```python
from build123d import *

# Parameters (mm, degrees)
PAD013_DEPTH    = 10
SKETCH065_W     = 4.5
SKETCH065_H     = 5.5
SKETCH065_W_2   = 3.4
SKETCH065_H_2   = 9
POCKET012_DEPTH = 7.2375310186


with BuildPart() as part:
    # Sketch064 → Pad013 (new body, symmetric)
    with BuildSketch(Plane.YZ):
        with BuildLine():
            ThreePointArc((-25.8475912574, 5.4708262373), (-29.159051684, -0.0593501339), (-30.5394960729, -6.355618405))
            ThreePointArc((-30.5394960729, -6.355618405), (-30.457390957, -6.658226438), (-30.2112344729, -6.8524424441))
            Line((-30.2112344729, -6.8524424441), (-29.3637121644, -7.1609153372))
            ThreePointArc((-29.3637121644, -7.1609153372), (-28.0255949556, -7.1024918781), (-27.1207148272, -6.1149885016))
            Line((-27.1207148272, -6.1149885016), (-23.4782003008, 3.8927379097))
            ThreePointArc((-23.4782003008, 3.8927379097), (-23.5115851346, 4.6573763148), (-24.0758727783, 5.1744506738))
            Line((-25.2946071344, 5.618033703), (-24.0758727783, 5.1744506738))
            ThreePointArc((-25.2946071344, 5.618033703), (-25.5942405308, 5.6313602812), (-25.8475912574, 5.4708262373))
        make_face()
    extrude(amount=PAD013_DEPTH, both=True)

    # Sketch065 (on Face6 of Pad013) → Pocket012 (cut, through all)
    with BuildSketch(Plane(origin=(0, -21.9828744359, 8.0011119583), x_dir=(0, 0.3420201433, 0.9396926208), z_dir=(0, 0.9396926208, -0.3420201433))):
        with Locations((-14.5220403435, 7.25)):
            Rectangle(SKETCH065_W, SKETCH065_H)
        with Locations((-14.5220403435, -7.25)):
            Rectangle(SKETCH065_W, SKETCH065_H)
        with Locations((-5.0720403435, 0)):
            Rectangle(SKETCH065_W_2, SKETCH065_H_2)
    extrude(amount=-POCKET012_DEPTH, mode=Mode.SUBTRACT)

    # SubtractivePipe003: sweep along a path in Sketch067
    with BuildLine(Plane.YZ.offset(4.5)) as subtractivepipe003_path:
        ThreePointArc((-25.6193920552, 5.7362457467), (-29.1630396012, -0.0694100418), (-30.5561005443, -6.7269214592))
    # Sketch066 (on DatumPlane) → SubtractivePipe003 (sweep, cut)
    with BuildSketch(Plane(origin=(4.5, -30.5394960729, -6.355618405), x_dir=(0, -0.9985433434, 0.0539554573), z_dir=(0, -0.0539554573, -0.9985433434))):
        Polygon((0, -0.025), (0, 0.025), (-0.0433012702, 0), align=None)
    subtractivepipe003 = sweep(path=subtractivepipe003_path.line, mode=Mode.SUBTRACT)

    # Mirrored003: SubtractivePipe003 across YZ
    add(subtractivepipe003.mirror(Plane.YZ), mode=Mode.SUBTRACT)


solid = part.part
```
Check sheet for the modelled part. Datum: model origin and axes. Units: mm. A direction names the side the tool comes from. Round coordinates to 2 decimals unless told otherwise and drop trailing zeros. Order: outer loops, then holes, each group sorted by start corner. A loop starts at its lowest first (then second) coordinate and runs counter-clockwise, first axis right, second up. Notation, with made-up numbers: (62.25, 44.5) - (117.25, 44.5) arc R9 ccw to (117.25, 60.5) - close; hole circle Ø6 at (-35, -22.5). An arc over 180 degrees is marked (long way). Answer as CSV lines item,"result". Start each with the question number.
1) Section check C-C (x = 4). Record the cut outline in (y, z), then the cut area to 3 significant figures.
2) Scan lines: probe 1 along X at (y, z) = (-25.5, 2.75); probe 2 along X at (y, z) = (-28.25, -3); probe 3 along Y at (x, z) = (-6.5, 3). Record each from-to range of solid material in increasing order.
3) Section check B-B (y = -24.75). Record the cut outline in (x, z).
4) Tool access check on faces 4 (the face through (4.5, -29, -5)), 5 (the face through (-4.5, -29, -5)), 6 (the face through (4.5, -25, 4)), 7 (the face through (-7.224, -28.249, 1.915)). Record the directions out of +Z, -Z, +X, -X, +Y, -Y that give a thin tool (end or side, any length) a straight path to the whole face; none if there is none.
5) Draft check along X on faces 1 (the face through (-0.06, -25.98, 2.25)), 2 (the face through (0.06, -28.04, -7.11)), 3 (the face through (-10, -27, 1)). Enter one of: +X half, -X half, draft (parallel to the pull), parting line (faces both ways), or undercut.
6) Section check A-A (x = 6.5). Record the cut outline in (y, z).
7) Depth check by flat-ended pin: pin 1 (4 mm diameter, centred on y = -28.5, z = -5.5, fed in from +X); pin 2 (2 mm diameter, centred on x = 2.5, y = -26.5, fed in from -Z); pin 3 (5 mm diameter, centred on x = -4.5, z = 1, fed in from +Y). Enter the tip coordinate at first touch or a pass-through.
Determined:
1,outline,"(-30.54, -6.36) arc R0.5 ccw to (-30.21, -6.85) - (-29.36, -7.16) arc R1.75 ccw to (-27.12, -6.11) - (-24.3, 1.64) - (-27.71, 2.88) arc R20 ccw to start"
1,area,"36.8 mm^2"
2,probe 1,"-10 to -4.5, 4.5 to 10"
2,probe 2,"-4.5 to 4.5"
2,probe 3,"-27.63 to -23.8"
3,outline,"(-10, 0.4) - (10, 0.4) - (10, 5.42) - (4.5, 5.42) - (4.5, 1.8) - (-4.5, 1.8) - (-4.5, 5.42) - (-10, 5.42) - close"
4,face 4,"-Z, +X, -Y"
4,face 5,"-Z, -X, -Y"
4,face 6,"+Z, +Y"
4,face 7,"+Z, +X, -X, -Y"
5,face 1,"undercut"
5,face 2,"draft"
5,face 3,"-X half"
6,outline,"(-29.87, -2.19) - (-26.18, -3.53) - (-23.48, 3.89) arc R1 ccw to (-24.08, 5.17) - (-25.29, 5.62) arc R0.5 ccw to (-25.85, 5.47) arc R20 ccw to start"
7,pin 1,"x = 4.5"
7,pin 2,"z = -6.73"
7,pin 3,"y = -23.62"
